from build123d import *

# Parameters (mm, degrees)
BOSS_EXTRUDE1_DEPTH = 8
SKETCH2_R           = 1.65
CUT_EXTRUDE1_DEPTH  = 24.597050759
SKETCH3_R           = 3
CUT_EXTRUDE2_DEPTH  = 2.3
SKETCH4_W           = 7.68
SKETCH4_H           = 8
SKETCH4_R           = 1.65
BOSS_EXTRUDE2_DEPTH = 18.5
FILLET1_R           = 5
CHAMFER1_SIZE       = 0.5


with BuildPart() as part:
    # Sketch1 → Boss-Extrude1 (new body)
    with BuildSketch(Plane.XY):
        with BuildLine():
            Line((0, 8), (15.38898322, 8))
            Line((15.38898322, 8), (15.38898322, 3.5))
            Line((15.38898322, 3.5), (2.321637353, 3.5))
            ThreePointArc((2.321637353, 3.5), (-4.2, 0), (2.321637353, -3.5))
            Line((2.321637353, -3.5), (15.38898322, -3.5))
            Line((15.38898322, -3.5), (15.38898322, -8))
            Line((15.38898322, -8), (0, -8))
            ThreePointArc((0, -8), (-8, 0), (0, 8))
        make_face()
    extrude(amount=BOSS_EXTRUDE1_DEPTH)

    # Sketch2 → Cut-Extrude1 (cut, through all)
    with BuildSketch(Plane.XZ.offset(8)):
        with Locations(Location((11.54898322, 4, 0), (0, 0, 270))):
            Circle(SKETCH2_R)
    extrude(amount=-CUT_EXTRUDE1_DEPTH, mode=Mode.SUBTRACT)

    # Sketch3 → Cut-Extrude2 (cut)
    with BuildSketch(Plane.XZ.offset(8)):
        with Locations(Location((11.54898322, 4, 0), (0, 0, 270))):
            Circle(SKETCH3_R)
    extrude(amount=-CUT_EXTRUDE2_DEPTH, mode=Mode.SUBTRACT)

    # Sketch4 → Boss-Extrude2 (add)
    with BuildSketch(Plane.XZ.offset(-3.5)):
        with Locations((11.54898322, 4)):
            Rectangle(SKETCH4_W, SKETCH4_H)
        with Locations(Location((11.54898322, 4, 0), (0, 0, 270))):
            Circle(SKETCH4_R, mode=Mode.SUBTRACT)
    extrude(amount=-BOSS_EXTRUDE2_DEPTH)

    # Fillet1
    fillet1_edges = [part.edges().sort_by_distance(p)[0] for p in [
        (7.70898322, 8, 4),
    ]]
    fillet(fillet1_edges, radius=FILLET1_R)

    # Chamfer1
    chamfer1_edges = [part.edges().sort_by_distance(p)[0] for p in [
        (8.855310287, 3.5, 0),
        (-4.2, 0, 0),
        (11.54898322, 22, 0),
        (7.70898322, 17.5, 0),
        (1.35449161, 8, 0),
        (6.244517126, 9.464466094, 0),
        (8.855310287, -3.5, 0),
        (15.38898322, -5.75, 0),
        (7.69449161, -8, 0),
        (-8, 0, 0),
        (15.38898322, 12.75, 0),
    ]]
    chamfer(chamfer1_edges, length=CHAMFER1_SIZE)


solid = part.part
Here's how the part is built. I have some questions about the finished solid (model axes, mm). A direction names the side the tool comes from. Round coordinates to 2 decimals unless told otherwise and drop trailing zeros. Loops run counter-clockwise (first coordinate to the right, second up) from the corner with the lowest first, then second, coordinate; pieces in that order, holes last.
1. We'd pull the mould along X, two halves only. Please class faces 4 (the face through (-4.333, 0.131, 0.365)), 5 (the face through (1, 8, 4)), 6 (the face through (-8, 0, 4)): +X half, -X half, draft (parallel to the pull), parting line (faces both ways), or undercut.
Answer list:
face 4: undercut
face 5: draft
face 6: -X half
2. If we section it at B-B on y = 17.25: Write out the boundary of the cut face in (x, z), plus the area to 3 significant figures.
Answer list:
outline: (7.71, 0.5) - (8.21, 0) - (14.89, 0) - (15.39, 0.5) - (15.39, 8) - (7.71, 8) - close; hole circle Ø3.3 at (11.55, 4)
area: 52.6 mm2
3. If we section it at C-C on y = 0: Write out the boundary of the cut face in (x, z), plus the area to 4 significant figures.
Answer list:
outline: (-8, 0.5) - (-7.5, 0) - (-4.7, 0) - (-4.2, 0.5) - (-4.2, 8) - (-8, 8) - close
area: 30.15 mm2
4. If I drill on line 1 along Y through (x, z) = (5, 3); line 2 along Z through (x, y) = (11.5, 5); line 3 along Y through (x, z) = (0, 2.25), over which ranges is the centre line in solid material (lowest first)?
Answer list:
line 1: y = -8 to -3.5, 3.5 to 8.56
line 2: z = 0 to 2.35, 5.65 to 8
line 3: y = -8 to -4.2, 4.2 to 8
5. If we section it at A-A on z = 4: Write out the boundary of the cut face in (x, y), plus the area to 3 significant figures.
Answer list:
outline: (0, -8) - (8.55, -8) - (8.55, -5.7) - (9.9, -5.7) - (9.9, -3.5) - (2.32, -3.5) arc R4.2 cw (long way) to (2.32, 3.5) - (9.9, 3.5) - (9.9, 22) - (7.71, 22) - (7.71, 13) arc R5 cw to (2.71, 8) - (0, 8) arc R8 ccw to start; (13.2, -5.7) - (14.55, -5.7) - (14.55, -8) - (15.39, -8) - (15.39, -3.5) - (13.2, -3.5) - close; (13.2, 3.5) - (15.39, 3.5) - (15.39, 22) - (13.2, 22) - close
area: 240 mm2
6. For P1, Ø2, axis at y = 16, z = 4.5, coming from the -X side; P2, Ø6.5, axis at x = 0, y = 0, coming from the -Z side; P3, Ø0.8, axis at x = 1, z = 4, coming from the +Y side, each with a flat end and sliding along its axis, tell me the tip position at first contact or that it passes through.
Answer list:
P1: stops at x = 7.71
P2: passes through
P3: stops at y = 8
7. Which directions (+Z, -Z, +X, -X, +Y, -Y) give clear straight access to the entire face, cutting with the end or side of a thin tool? Please do faces 1 (the face through (8.62, -6.87, 4.65)), 2 (the face through (9, 3.5, 4)), 3 (the face through (7.709, 17, 4)).
Answer list:
face 1: -Y
face 2: +Z, -Z, +X
face 3: +Z, -Z, -X, +Y
